Autodesk Fusion 360 part; units mm, degrees
sketch "スケッチ1" plane through (0, 0, 0) normal (0, 0, 1) x (1, 0, 0)
  line L0 (0, 0) -> (286.75, 0)
  line L1 (286.75, 0) -> (286.75, -96.25)
  line L2 (286.75, -96.25) -> (0, -96.25)
  line L3 (0, -96.25) -> (0, 0)
  line L4 (-15, 10) -> (301.75, 10)
  line L5 (301.75, 10) -> (301.75, -106.25)
  line L6 (301.75, -106.25) -> (-15, -106.25)
  line L7 (-15, -106.25) -> (-15, 10)
  circle A0 centre (260.95, -28.5) radius 2
  circle A1 centre (282.75, -57.25) radius 2
  circle A2 centre (191.45, -85.85) radius 2
  circle A3 centre (4, -57.25) radius 2
  circle A4 centre (26, -28.5) radius 2
  line L8 (286.75, -59.25) -> (282.75, -59.25)
  line L9 (286.75, -55.25) -> (282.75, -55.25)
  line L10 (0, -59.25) -> (4, -59.25)
  line L11 (0, -55.25) -> (4, -55.25)
  circle A5 centre (129, -47.75) radius 2
  circle A6 centre (4, -57.25) radius 0.9
  circle A7 centre (26, -28.5) radius 0.9
  circle A8 centre (191.45, -85.85) radius 0.9
  circle A9 centre (129, -47.75) radius 0.9
  circle A10 centre (282.75, -57.25) radius 0.9
  circle A11 centre (260.95, -28.5) radius 0.9
  dimension "d7" = 286.75
  dimension "d8" = 96.25
  dimension "d9" = 15
  dimension "d10" = 10
  dimension "d11" = 10
  dimension "d12" = 15
  dimension "d13" = 4
  dimension "d14" = 28.5
  dimension "d15" = 25.8
  dimension "d16" = 4
  dimension "d17" = 4
  dimension "d18" = 4
  dimension "d19" = 4
  dimension "d20" = 28.5
  dimension "d21" = 26
  dimension "d22" = 39
  dimension "d23" = 4
  dimension "d24" = 4
  dimension "d25" = 39
  dimension "d26" = 10.4
  dimension "d27" = 95.3
  dimension "d28" = 4
  dimension "d29" = 129
  dimension "d30" = 48.5
  dimension "d54" = 1.8
  dimension "d55" = 1.8
  dimension "d56" = 1.8
  dimension "d57" = 1.8
  dimension "d58" = 1.8
  dimension "d59" = 1.8
extrude "押し出し1" add sketch "スケッチ1" along normal blind 14.1 contours L4 L5 L6 L7
extrude "押し出し2" add sketch "スケッチ1" against normal blind 4 contours L4 L5 L6 L7
sketch "スケッチ2" plane through (0, 0, -4) normal (0, 0, -1) x (1, 0, 0)
  line L0 (0, 96.25) -> (286.75, 96.25)
  line L1 (286.75, 96.25) -> (286.75, 0)
  line L2 (286.75, 0) -> (0, 0)
  line L3 (0, 0) -> (0, 96.25)
  line L4 (301.75, 106.25) -> (-15, 106.25)
  line L5 (-15, 106.25) -> (-15, -10)
  line L6 (-15, -10) -> (301.75, -10)
  line L7 (301.75, -10) -> (301.75, 106.25)
extrude "押し出し3" add sketch "スケッチ2" along normal blind 15 contours L0 L1 L2 L3 | L4 L5 L6 L7
sketch "スケッチ3" plane through (-15, 0, 0) normal (-1, 0, 0) x (0, -1, 0)
  line L0 (106.25, -19) -> (106.25, 14.1)
  line L1 (106.25, 14.1) -> (-10, 14.1)
  line L2 (-10, 14.1) -> (-10, -19)
  line L3 (-10, -19) -> (106.25, -19)
  line L4 (-10, -19) -> (106.25, -4.7263)
  line L5 (3.7947, -17.3062) -> (-10, 1)
  dimension "d37" = 7
  dimension "d77" = 120
  dimension "d78" = 20
extrude "押し出し4" cut sketch "スケッチ3" against normal blind 320 contours L0 L3 L4 | L2 L4 L5
extrude "押し出し5" add sketch "スケッチ1" against normal blind 4 contours L3 A3 L10 L11 | L1 A1 L8 L9 | A3 | A1 | A0 | A2 | A4 | A6 | A7 | A8 | A10 | A11
sketch "スケッチ4" plane through (0, 10, 0) normal (0, 1, 0) x (-1, 0, 0)
  line L0 (15, 1) -> (15, 14.1)
  line L1 (15, 14.1) -> (-301.75, 14.1)
  line L2 (-301.75, 14.1) -> (-301.75, 1)
  line L3 (-29, 4.6) -> (-9, 4.6)
  line L4 (-9, 4.6) -> (-9, -9.4)
  line L5 (-9, -9.4) -> (-29, -9.4)
  line L6 (-29, -9.4) -> (-29, 4.6)
  line L7 (-26, -0.4) -> (-12, -0.4)
  line L8 (-12, -0.4) -> (-12, -4.4)
  line L9 (-12, -4.4) -> (-26, -4.4)
  line L10 (-26, -4.4) -> (-26, -0.4)
  line L11 (-301.75, 1) -> (15, 1)
  dimension "d42" = 20
  dimension "d43" = 14
  dimension "d44" = 24
  dimension "d45" = 9.5
  dimension "d46" = 14
  dimension "d47" = 4
  dimension "d48" = 27
  dimension "d49" = 14.5
extrude "押し出し6" cut sketch "スケッチ4" against normal blind 20 contours L7 L8 L9 L10
extrude "押し出し7" cut sketch "スケッチ4" against normal blind 8 contours L3 L4 L6 L11 | L4 L5 L6 L11
extrude "押し出し8" cut sketch "スケッチ1" against normal blind 5 contours A6 | A7 | A8 | A10 | A11
sketch "スケッチ6" plane through (-15, 0, 0) normal (-1, 0, 0) x (0, -1, 0)
  line L0 (3.7947, -17.3062) -> (106.25, -4.7263)
  line L1 (106.25, 14.1) -> (-10, 14.1)
  line L2 (-10, 1) -> (26.6233, -14.5032)
  line L3 (-10, 1) -> (50.4444, -11.5784)
  line L4 (-10, 1) -> (106.25, -4.7263)
  line L5 (-10, 1) -> (74.2655, -8.6535)
  line L6 (-10, 1) -> (3.7947, -17.3062)
  line L7 (106.25, -4.7263) -> (106.25, 14.1)
  line L8 (-10, 14.1) -> (-10, 1)
  point P0 (-10, 1)
  dimension "d79" = 23
  dimension "d80" = 47
  dimension "d81" = 71
  dimension "d82" = 103.2247
sketch "スケッチ7" plane through (0, 10, 0) normal (0, 1, 0) x (-1, 0, 0)
  line L0 (-29, 4.6) -> (-9, 4.6)
  line L1 (-9, 1) -> (15, 1)
  line L2 (15, 14.1) -> (-301.75, 14.1)
  line L3 (15, 1) -> (10, 1)
  line L4 (10, 1) -> (10, -24)
  line L5 (10, -24) -> (15, -24)
  line L6 (15, -24) -> (15, 1)
  line L7 (10, 1) -> (7.5, 1)
  line L8 (7.5, 1) -> (7.5, -24)
  line L9 (7.5, -24) -> (10, -24)
  line L10 (10, -24) -> (10, 1)
  line L11 (7.5, 1) -> (5, 1)
  line L12 (5, 1) -> (5, -24)
  line L13 (5, -24) -> (7.5, -24)
  line L14 (7.5, -24) -> (7.5, 1)
  line L15 (5, 1) -> (2.5, 1)
  line L16 (2.5, 1) -> (2.5, -24)
  line L17 (2.5, -24) -> (5, -24)
  line L18 (5, -24) -> (5, 1)
  line L19 (15, 1) -> (15, 14.1)
  line L20 (-301.75, 14.1) -> (-301.75, 1)
  line L21 (-9, 4.6) -> (-9, 1)
  line L22 (-301.75, 1) -> (-29, 1)
  line L23 (-29, 1) -> (-29, 4.6)
  dimension "d83" = 25
  dimension "d84" = 5
  dimension "d85" = 2.5
  dimension "d86" = 25
  dimension "d87" = 2.5
  dimension "d88" = 25
  dimension "d89" = 2.5
  dimension "d90" = 25
sweep "スイープ1" cut profiles "スケッチ7" path "スケッチ6" along L4 section 1 contours L1 L3 L4 L5 L6 L10
sweep "スイープ2" cut profiles "スケッチ7" path "スケッチ6" along L5 section 1 contours L1 L4 L7 L8 L9 L10 L14
sweep "スイープ3" cut profiles "スケッチ7" path "スケッチ6" along L3 section 1 contours L1 L8 L11 L12 L13 L14 L18
sweep "スイープ4" cut profiles "スケッチ7" path "スケッチ6" along L2 section 1 contours L1 L12 L15 L16 L17 L18
sketch "スケッチ8" plane through (301.75, 0, 0) normal (1, 0, 0) x (0, 1, 0)
  line L0 (-106.25, -4.7263) -> (-3.7947, -17.3062)
  line L1 (-3.7947, -17.3062) -> (10, 1)
  line L2 (10, 1) -> (10, 14.1)
  line L3 (10, 14.1) -> (-106.25, 14.1)
  line L4 (-106.25, 14.1) -> (-106.25, -4.7263)
  line L5 (10, 1) -> (-106.25, -4.7263)
  line L6 (10, 1) -> (-74.2655, -8.6535)
  line L7 (10, 1) -> (-50.4444, -11.5784)
  line L8 (10, 1) -> (-26.6233, -14.5032)
  dimension "d116" = 23
  dimension "d117" = 47
  dimension "d118" = 71
sketch "スケッチ9" plane through (0, 10, 0) normal (0, 1, 0) x (-1, 0, 0)
  line L0 (-9, 1) -> (2.5, 1)
  line L1 (15, 1) -> (15, 14.1)
  line L2 (15, 14.1) -> (-301.75, 14.1)
  line L3 (-301.75, 14.1) -> (-301.75, 1)
  line L4 (-301.75, 1) -> (-29, 1)
  line L5 (-29, 4.6) -> (-9, 4.6)
  line L6 (-301.75, 1) -> (-296.75, 1)
  line L7 (-296.75, 1) -> (-296.75, -24)
  line L8 (-296.75, -24) -> (-301.75, -24)
  line L9 (-301.75, -24) -> (-301.75, 1)
  line L10 (-296.75, 1) -> (-294.25, 1)
  line L11 (-294.25, 1) -> (-294.25, -24)
  line L12 (-294.25, -24) -> (-296.75, -24)
  line L13 (-296.75, -24) -> (-296.75, 1)
  line L14 (-294.25, 1) -> (-291.75, 1)
  line L15 (-291.75, 1) -> (-291.75, -24)
  line L16 (-291.75, -24) -> (-294.25, -24)
  line L17 (-294.25, -24) -> (-294.25, 1)
  line L18 (-291.75, 1) -> (-289.25, 1)
  line L19 (-289.25, 1) -> (-289.25, -24)
  line L20 (-289.25, -24) -> (-291.75, -24)
  line L21 (-291.75, -24) -> (-291.75, 1)
  line L22 (-9, 4.6) -> (-9, 1)
  line L23 (2.5, 1) -> (5, 1)
  line L24 (5, 1) -> (7.5, 1)
  line L25 (7.5, 1) -> (10, 1)
  line L26 (10, 1) -> (15, 1)
  line L27 (-29, 1) -> (-29, 4.6)
  dimension "d119" = 5
  dimension "d120" = 25
  dimension "d121" = 2.5
  dimension "d122" = 25
  dimension "d123" = 2.5
  dimension "d124" = 25
  dimension "d125" = 2.5
  dimension "d126" = 25
sweep "スイープ5" cut profiles "スケッチ9" path "スケッチ8" along L5 section 1 contours L4 L6 L7 L8 L9 L13
sweep "スイープ6" cut profiles "スケッチ9" path "スケッチ8" along L6 section 1 contours L4 L7 L10 L11 L12 L13 L17
sweep "スイープ7" cut profiles "スケッチ9" path "スケッチ8" along L7 section 1 contours L4 L11 L14 L15 L16 L17 L21
sweep "スイープ8" cut profiles "スケッチ9" path "スケッチ8" along L8 section 1 contours L4 L15 L18 L19 L20 L21
fillet "フィレット6" radius 2 4 edges at (0, 0, 5.05) (0, -96.25, 5.05) (286.75, -96.25, 5.05) (286.75, 0, 5.05)
sketch "スケッチ11" plane through (0, 0, 14.1) normal (0, 0, 1) x (-1, 0, 0)
  line L0 (-284.75, 96.25) -> (-2, 96.25)
  arc A0 (0, 94.25) -> (-2, 96.25) centre (-2, 94.25) ccw
  line L1 (0, 94.25) -> (0, 2)
  arc A1 (-2, 0) -> (0, 2) centre (-2, 2) ccw
  line L2 (-2, 0) -> (-284.75, 0)
  arc A2 (-286.75, 2) -> (-284.75, 0) centre (-284.75, 2) ccw
  line L3 (-286.75, 2) -> (-286.75, 94.25)
  arc A3 (-284.75, 96.25) -> (-286.75, 94.25) centre (-284.75, 94.25) ccw
  line L4 (15, 106.25) -> (-301.75, 106.25)
  line L5 (-301.75, 106.25) -> (-301.75, -10)
  line L6 (-301.75, -10) -> (15, -10)
  line L7 (15, -10) -> (15, 106.25)
  line L8 (0, 0) -> (-286.75, 0)
  line L9 (-286.75, 0) -> (-286.75, 96.25)
  line L10 (-286.75, 96.25) -> (0, 96.25)
  line L11 (0, 96.25) -> (0, 0)
extrude "押し出し11" cut sketch "スケッチ11" against normal blind 9 contours A3 L9 L10 | A0 L10 L11 | A2 L8 L9 | A1 L8 L11
fillet "フィレット7" radius 1 4 edges at (286.75, 0, 9.6) (286.75, -96.25, 9.6) (0, -96.25, 9.6) (0, 0, 9.6)
fillet "フィレット5" radius 5 4 edges at (9, 6, 4.6) (9, 2.0815, -9.4) (29, 2.0815, -9.4) (29, 6, 4.6)
chamfer "面取り2" distance 5 angle 45 4 edges at (301.75, -106.25, 4.6869) (301.75, 10, 7.55) (-15, 10, 7.55) (-15, -106.25, 4.6869)
chamfer "面取り3" distance 5 angle 45 4 edges at (301.75, -48.125, 14.1) (143.375, -106.25, 14.1) (143.375, 10, 14.1) (-15, -48.125, 14.1)
chamfer "面取り6" distance 0.5 angle 45 1 edges at (301.75, -48.125, -1.8631)
chamfer "面取り6" distance 0.1 angle 45 7 edges at (9, 7.4379, -2.4) (9.0503, 9.4779, 0.3071) (28.9497, 9.4779, 0.3071) (29, 7.4379, -2.4) (27.5355, 3.2666, -7.9355) (19, 2.163, -9.4) (10.4645, 3.2666, -7.9355)
chamfer "面取り6" distance 1 angle 45 3 edges at (11, 10, 3.6) (27, 10, 3.6) (19, 10, 4.6)
chamfer "面取り7" distance 0.5 angle 45 2 edges at (143.375, -3.7947, -17.3062) (143.375, -106.25, -4.7263)
equation "d7 = ( 19.05 * 15 ) * 1 mm + ( 0.5 * 2 ) * 1 mm"
equation "d8 = ( 19.05 * 5 ) * 1 mm + ( 0.5 * 2 ) * 1 mm"
equation "d14 = 28 mm + 0.5 mm"
equation "d15 = 25.3 mm + 0.5 mm"
equation "d20 = 28 mm + 0.5 mm"
equation "d21 = 25.5 mm + 0.5 mm"
equation "d22 = 38.5 mm + 0.5 mm"
equation "d23 = 3.5 mm + 0.5 mm"
equation "d24 = 3.5 mm + 0.5 mm"
equation "d25 = 38.5 mm + 0.5 mm"
equation "d26 = 9.9 mm + 0.5 mm"
equation "d27 = 94.8 mm + 0.5 mm"
equation "d29 = 128.5 mm + 0.5 mm"
equation "d30 = 48 mm + 0.5 mm"
equation "d31 = 7.5 mm + 5 mm + 1.6 mm"
equation "d33 = -2 mm - 2 mm"
equation "d44 = 9 mm + 15 mm"
equation "d48 = 12 mm + 15 mm"
equation "d80 = ( 23 * 2 ) * 1 mm + 1 mm"
equation "d81 = ( 23 * 3 ) * 1 mm + 2 mm"
equation "d117 = ( 23 * 2 ) * 1 mm + 1 mm"
equation "d118 = ( 23 * 3 ) * 1 mm + 2 mm"
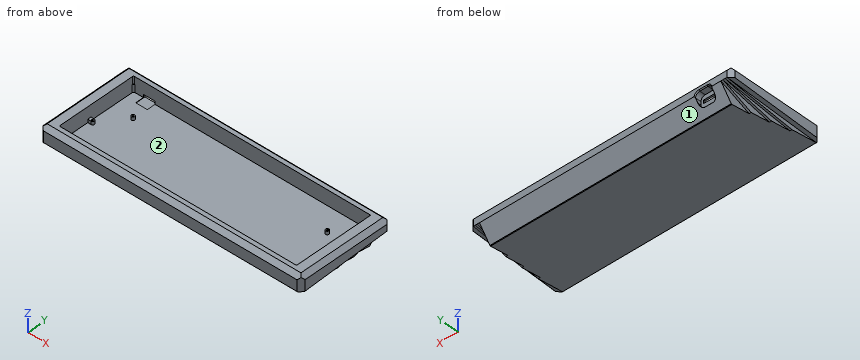
Could you check a few things on this model? Use its own coordinates, in mm. Face numbers are marked on the shaded views. Coordinates: 2 decimals unless noted, no trailing zeros. Order: outer loops, then holes, each group sorted by start corner. A loop starts at its lowest first (then second) coordinate and runs counter-clockwise, first axis right, second up. Notation, with made-up numbers: M 33.5,25 L 59.5,25 A25 ccw 59.5,59 Z; hole C -18.75,80 d3. An arc over 180 degrees is marked long. Use one line per item in the form item = value. Start each with the question number.
1. Suppose I cut it at B-B on y = -13.5. Write out the boundary of the cut face in (x, z), then the cut area to 3 significant figures.
2. We'd pull the mould along X, two halves only. Please class the marked faces 1 and 2: +X half, -X half, draft (parallel to the pull), parting line (faces both ways), or undercut.
3. For pin 1 (1.4 mm diameter, centred on x = 260.95, y = -28.5, fed in from +Z); pin 2 (2 mm diameter, centred on y = 5.5, z = -2.5, fed in from +X); pin 3 (1.2 mm diameter, centred on x = 2, z = -1, fed in from +Y) (3 decimals), each with a flat end and sliding along its axis, tell me the tip position at first contact or that it passes through.
4. Please list where these lines run through material, in increasing order: line 1 (X direction, y = -57.25, z = -2.5); line 2 (X direction, y = -57.25, z = -1.4); line 3 (X direction, y = -52, z = 9).
5. Suppose I cut it at A-A on x = 62. Write out the boundary of the cut face in (y, z), then the cut area to 3 significant figures.
Geometry says:
q1.outline = M -15,-0.16 L -10,-0.16 L -10,-1.69 L -7.5,-1.69 L -7.5,-3.89 L -5,-3.89 L -5,-8.95 L -2.5,-8.95 L -2.5,-16.11 L 289.25,-16.11 L 289.25,-8.95 L 291.75,-8.95 L 291.75,-3.89 L 294.25,-3.89 L 294.25,-1.69 L 296.75,-1.69 L 296.75,-0.16 L 301.25,-0.16 L 301.75,0.34 L 301.75,9.1 L 296.75,14.1 L 286.75,14.1 L 286.75,-4 L 0,-4 L 0,14.1 L -10,14.1 L -15,9.1 Z
q1.area = 4,030 mm^2
q2.face_1 = draft
q2.face_2 = undercut
q3.pin_1 = -5
q3.pin_2 = 289.25
q3.pin_3 = 8.945
q4.line_1 = -10 to 3.1, 4.9 to 6, 280.75 to 281.85, 283.65 to 296.75
q4.line_2 = -15 to 3.1, 4.9 to 6, 280.75 to 281.85, 283.65 to 301.75
q4.line_3 = -15 to 0, 286.75 to 301.75
q5.outline = M -106.25,-4.23 L -105.75,-4.79 L -4.29,-17.25 L -3.49,-16.91 L 10,1 L 10,9.1 L 5,14.1 L 0,14.1 L 0,-4 L -96.25,-4 L -96.25,14.1 L -101.25,14.1 L -106.25,9.1 Z
q5.area = 1,110 mm^2
